Autodesk Inventor part; units mm, degrees
ref_plane "YZ Plane" through (0, 0, 0) normal (1, 0, 0) x (0, 1, 0)
ref_plane "XZ Plane" through (0, 0, 0) normal (0, 1, 0) x (-1, 0, 0)
ref_plane "XY Plane" through (0, 0, 0) normal (0, 0, 1) x (1, 0, 0)
sketch "Sketch1" plane through (0, 0, 0) normal (0, 0, 1) x (1, 0, 0)
  line L0 (-1.0414, 0) -> (6.2484, 0) construction
  line L1 (0, -0.3556) -> (0, 2.1336) construction
  line L2 (1.651, 0) -> (5.207, 0)
  line L3 (5.207, 0) -> (5.207, 1.778)
  line L4 (5.207, 1.778) -> (4.572, 1.778)
  line L5 (4.572, 1.778) -> (4.5189, 1.143)
  line L6 (4.5189, 1.143) -> (4.7625, 1.143)
  line L7 (4.7625, 1.143) -> (4.7625, 0.508)
  line L8 (4.7625, 0.508) -> (1.651, 0.508)
  line L9 (1.651, 0.508) -> (1.651, 0)
  point P0 (0, 0)
  dimension "d0" = 3.302
  dimension "d1" = 10.414
  dimension "d2" = 1.778
  dimension "d3" = 0.635
  dimension "d4" = 9.0378
  dimension "d5" = 9.525
  dimension "d6" = 0.508
  dimension "d7" = 0.635
revolve "Revolution1" add sketch "Sketch1" angle 360 about axis through (0, -10, 0) along (0, 1, 0)
fillet "Fillet1" radius 0.381 1 edges at (-5.207, 0, 0)
fillet "Fillet2" radius 0.127 3 edges at (-5.207, 1.778, 0) (-4.572, 1.778, 0) (-4.7625, 0.508, 0)
equation "\"d7\" = d3"
properties part number "Shock Cartridge Cover"
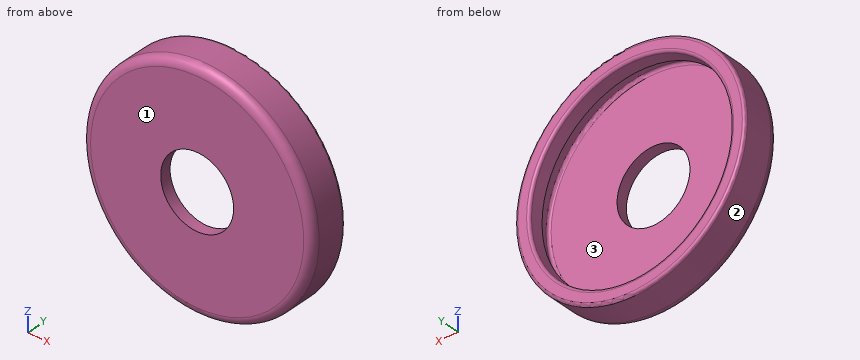
The model under review builds one solid part; all positions refer to its coordinate system, in mm. Face numbers are marked on the shaded views. Round coordinates to 2 decimals unless told otherwise and drop trailing zeros. Loops run counter-clockwise (first coordinate to the right, second up) from the corner with the lowest first, then second, coordinate; pieces in that order, holes last. Notation, with made-up numbers: (84.25, -11.75) -> (98.25, -11.75) arc R34 ccw to (98.25, 25.25) -> close; hole circle Ø8 at (-37.75, 72.5). An arc over 180 degrees is marked (long way). Answer as CSV lines item,"result".
1) For P1, Ø2, axis at x = 0, z = 0, coming from the +Y side; P2, Ø1, axis at x = -1.5, z = -1.5, coming from the +Y side, all flat-tipped, find the tip position at first contact; note any pin that passes through.
Geometry results:
P1,"passes through"
P2,"stops at y = 0.51"
2) Add section C-C on y = 1.3. Write out the cut boundary in (x, z), plus the area to 3 significant figures.
Geometry results:
outline,"circle Ø10.41 at (0, 0); hole circle Ø9.06 at (0, 0)"
area,"20.7 mm²"
3) Draft analysis for pull direction Z (two halves, no side actions). For the marked faces 1, 2 and 3, state which applies: pulls with the +Z half, pulls with the -Z half, needs draft (parallel to the pull), parting line crosses it, or undercut.
Geometry results:
face 1,"needs draft"
face 2,"parting line crosses it"
face 3,"undercut"
4) To check wall thickness, follow line 1 along Z through (x, y) = (0, 1.05); line 2 along X through (y, z) = (0.4, 0); line 3 along Y through (x, z) = (3.5, -0.5). State the ranges of each line that lie inside material, in increasing order. Write a range as from..to.
Geometry results:
line 1,"z = -5.21..-4.76, 4.76..5.21"
line 2,"x = -5.21..-1.65, 1.65..5.21"
line 3,"y = 0..0.51"
